Geometry: see drawing. Coordinates: mm, zero at the bounding-box minimum. A direction names the side the tool comes from. Round coordinates to 2 decimals unless told otherwise and drop trailing zeros. Order: outer loops, then holes, each group sorted by start corner. A loop starts at its lowest first (then second) coordinate and runs counter-clockwise, first axis right, second up. Notation, with made-up numbers: (-13.5, -13.5) - (40.5, -13.5) arc R10 ccw to (40.5, -1.5) - close; hole circle Ø11 at (42, 88). An arc over 180 degrees is marked (long way). Put each result on its own line as item: value. Start each with the question number.
1) Contact query for flat-ended pins moving along their axis: P1, Ø4, axis at x = 6, y = 5, coming from the -Z side; P2, Ø6.5, axis at x = 15, z = 6, coming from the -Y side. Output: stop coordinate, or through.
2) Line query: probe 1 along Y at (x, z) = (24, 6.75); probe 2 along X at (y, z) = (4, 9.5); probe 3 along Z at (x, y) = (15, 6.5). Output: solid intervals per line, ascending. Write a range as [from, to].
3) Section A-A on x = 15. Output: boundary loops of the cut face in (y, z), then the cut area to 3 significant figures.
4) Section B-B on z = 0.5. Output: boundary loops of the cut face in (x, y).
5) Section C-C on y = 5. Output: boundary loops of the cut face in (x, z), then the cut area to 3 significant figures.
6) Mould query, pull axis X, two halves, no side actions, for the marked faces 3, 4 and 5. Classes: +X half, -X half, draft (parallel to the pull), parting line (faces both ways), or undercut.
7) Access query for the marked faces 1 and 2. Directions: +Z, -Z, +X, -X, +Y, -Y. A direction counts if a zero-diameter tool reaches every point of the face in a straight line with its end or side. Return the directions, or none.
8) Section D-D on x = 6. Output: boundary loops of the cut face in (y, z).
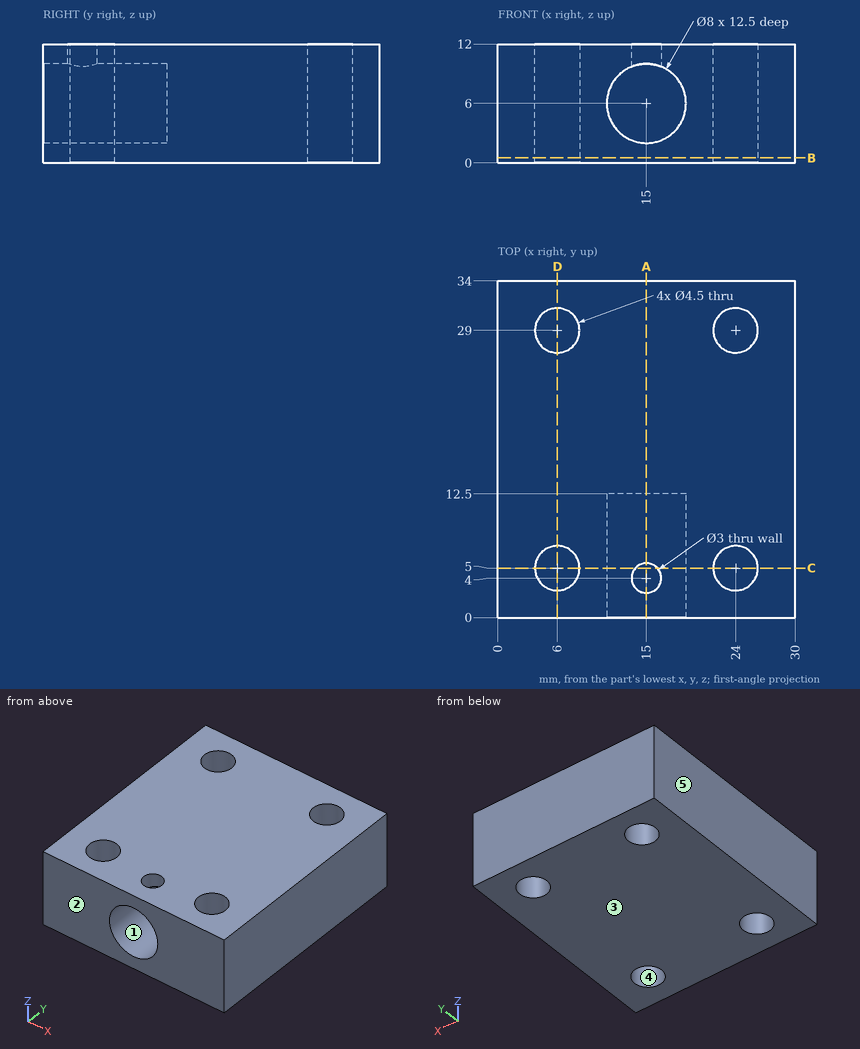
Answer sheet:
1. P1: through
1. P2: y = 12.5
2. probe 1: [0, 2.75], [7.25, 26.75], [31.25, 34]
2. probe 2: [0, 3.98], [8.02, 13.06], [16.94, 21.98], [26.02, 30]
2. probe 3: [0, 2], [10, 12]
3. outline: (0, 0) - (34, 0) - (34, 12) - (5.5, 12) - (5.5, 10) - (12.5, 10) - (12.5, 2) - (0, 2) - close; (0, 10) - (2.5, 10) - (2.5, 12) - (0, 12) - close
3. area: 302 mm^2
4. outline: (0, 0) - (30, 0) - (30, 34) - (0, 34) - close; hole circle Ø4.5 at (6, 5); hole circle Ø4.5 at (6, 29); hole circle Ø4.5 at (24, 5); hole circle Ø4.5 at (24, 29)
5. outline: (0, 0) - (3.75, 0) - (3.75, 12) - (0, 12) - close; (8.25, 0) - (21.75, 0) - (21.75, 12) - (16.12, 12) - (16.12, 9.84) arc R4 cw (long way) to (13.88, 9.84) - (13.88, 12) - (8.25, 12) - close; (26.25, 0) - (30, 0) - (30, 12) - (26.25, 12) - close
5. area: 197 mm^2
6. face 3: draft
6. face 4: undercut
6. face 5: -X half
7. face 1: -Y
7. face 2: +Z, -Z, +X, -X, -Y
8. outline: (0, 0) - (2.75, 0) - (2.75, 12) - (0, 12) - close; (7.25, 0) - (26.75, 0) - (26.75, 12) - (7.25, 12) - close; (31.25, 0) - (34, 0) - (34, 12) - (31.25, 12) - close
